Geometry check sheet. Reference: the model listing, model coordinates, mm. A direction names the side the tool comes from. Give positions to 0.01 mm unless a question says otherwise; leave off trailing zeros. Order: outer loops, then holes, each group sorted by start corner. A loop starts at its lowest first (then second) coordinate and runs counter-clockwise, first axis right, second up. Notation, with made-up numbers: (10.25, -11) - (42.25, -11) arc R19 cw to (42.25, 24) - close; hole circle Ø10 at (-32.5, 6). An arc over 180 degrees is marked (long way). Put each result on its own line as item: value. Start each with the question number.
```python
from build123d import *

# Parameters (mm, degrees)
F0_R           = 15
F1_DEPTH       = 30
F3_DEPTH       = 25
F3_DEPTH_BACK  = 25
F5_DEPTH       = 14
F6_R           = 5
F7_R           = 2
F8_DEPTH       = 25
F8_DEPTH_BACK  = 25
F9_R           = 1.25
F10_DEPTH      = 25
F10_DEPTH_BACK = 25


with BuildPart() as f1:
    # F0 (on Front) → F1 (new body)
    with BuildSketch(Plane.XZ):
        Circle(F0_R)
    extrude(amount=F1_DEPTH)

    # F2 (on Right) → F3 (cut, two sides)
    with BuildSketch(Plane.YZ) as f3_sk:
        with BuildLine():
            Line((15, 8), (-7, 8))
            ThreePointArc((-7, 8), (-12.6568542495, 5.6568542495), (-15, 0))
            ThreePointArc((-15, 0), (-12.6568542495, -5.6568542495), (-7, -8))
            Line((-7, -8), (15, -8))
            Line((15, -8), (15, 8))
        make_face()
    extrude(amount=-F3_DEPTH, mode=Mode.SUBTRACT)
    extrude(f3_sk.sketch, amount=F3_DEPTH_BACK, mode=Mode.SUBTRACT)

    # F4 (on face) → F5 (join)
    with BuildSketch(Plane.XZ.offset(30)):
        with BuildLine():
            ThreePointArc((13.7477270849, 0), (11.990367772, 4.2426406871), (7.7477270849, 6))
            Line((7.7477270849, 6), (-7.7477270849, 6))
            ThreePointArc((-7.7477270849, 6), (-11.990367772, 4.2426406871), (-13.7477270849, 0))
            ThreePointArc((-13.7477270849, 0), (-11.990367772, -4.2426406871), (-7.7477270849, -6))
            Line((-7.7477270849, -6), (7.7477270849, -6))
            ThreePointArc((7.7477270849, -6), (11.990367772, -4.2426406871), (13.7477270849, 0))
        make_face()
    extrude(amount=F5_DEPTH)

    # F6
    f6_edges = [f1.edges().sort_by_distance(p)[0] for p in [
        (13.747727, -44, 0),
        (0, -44, 6),
        (-13.747727, -44, 0),
        (0, -44, -6),
    ]]
    fillet(f6_edges, radius=F6_R)

    # F7 (on Top) → F8 (cut, two sides)
    with BuildSketch(Plane.XY) as f8_sk:
        with Locations((0, -35.9389074147)):
            Circle(F7_R)
    extrude(amount=-F8_DEPTH, mode=Mode.SUBTRACT)
    extrude(f8_sk.sketch, amount=F8_DEPTH_BACK, mode=Mode.SUBTRACT)

    # F9 (on Top) → F10 (cut, two sides)
    with BuildSketch(Plane.XY) as f10_sk:
        with Locations((0, -3.3346442506)):
            Circle(F9_R)
    extrude(amount=-F10_DEPTH, mode=Mode.SUBTRACT)
    extrude(f10_sk.sketch, amount=F10_DEPTH_BACK, mode=Mode.SUBTRACT)


solid = f1.part
```
Item 1: Gauge pin test, flat ends, axial feed: pin 1 Ø4.5 at (x, y) = (0, -35.94) entering from -Z; pin 2 Ø1.5 at (y, z) = (-39, -5.5) entering from +X; pin 3 Ø3 at (x, y) = (0, -35.94) entering from +Z; pin 4 Ø5 at (x, y) = (4.5, -6.5) entering from -Z. Record the tip position at first contact, or that the pin passes through.
Item 2: Cross-section at C-C (z = 11). Enter the section's corners in (x, y).
Item 3: Cross-section at D-D (x = 4). Enter the section's corners in (y, z).
Item 4: Set-up check for faces 1 (the face through (0, -33, -6)), 2 (the face through (0, -33, 6)), 3 (the face through (0.2, -1.9, 8)): record each of +Z, -Z, +X, -X, +Y, -Y from which the full face is reachable in a straight line by a thin tool's end or side.
Item 5: Release check for a two-part mould opening along X. For faces 4 (the face through (-14.985, -18.123, 0.66)), 5 (the face through (0, -42, -5)), 6 (the face through (-0.271, -4.555, -11.452)) record: +X half, -X half, draft (parallel to the pull), parting line (faces both ways), or undercut.
Item 6: Cross-section at B-B (y = -35). Enter the section's corners in (x, z), and give its area (3 significant figures).
Item 7: Thickness scan on line 1 along Y through (x, z) = (0, -11.5); line 2 along Y through (x, z) = (0, -1.85); line 3 along Z through (x, y) = (6, -13). Record the ranges inside material, lowest first.
Item 8: Cross-section at A-A (x = 0). Enter the section's corners in (y, z).
Recorded:
1. pin 1: stops at z = -6
1. pin 2: stops at x = 11.41
1. pin 3: passes through
1. pin 4: stops at z = -14.87
2. outline: (-10.2, -30) - (10.2, -30) - (10.2, 0) - (-10.2, 0) - close; hole circle Ø2.5 at (0, -3.33)
3. outline: (-44, -1) arc R5 ccw to (-39, -6) - (-30, -6) - (-30, -14.46) - (0, -14.46) - (0, -8) - (-7, -8) arc R8 cw to (-7, 8) - (0, 8) - (0, 14.46) - (-30, 14.46) - (-30, 6) - (-39, 6) arc R5 ccw to (-44, 1) - close
4. face 1: -Z, +X, -X, -Y
4. face 2: +Z, +X, -X, -Y
4. face 3: +X, -X, +Y
5. face 4: parting line
5. face 5: draft
5. face 6: undercut
6. outline: (-7.75, -6) - (-1.77, -6) - (-1.77, 6) - (-7.75, 6) arc R6 ccw to start; (1.77, -6) - (7.75, -6) arc R6 ccw to (7.75, 6) - (1.77, 6) - close
6. area: 257 mm^2
7. line 1: y = -30 to -4.58, -2.08 to 0
7. line 2: y = -43.93 to -37.94, -33.94 to -14.78
7. line 3: z = -13.75 to -5.29, 5.29 to 13.75
8. outline: (-44, -1) arc R5 ccw to (-39, -6) - (-37.94, -6) - (-37.94, 6) - (-39, 6) arc R5 ccw to (-44, 1) - close; (-33.94, -6) - (-30, -6) - (-30, -15) - (-4.58, -15) - (-4.58, -8) - (-7, -8) arc R8 cw to (-7, 8) - (-4.58, 8) - (-4.58, 15) - (-30, 15) - (-30, 6) - (-33.94, 6) - close; (-2.08, -15) - (0, -15) - (0, -8) - (-2.08, -8) - close; (-2.08, 8) - (0, 8) - (0, 15) - (-2.08, 15) - close
